Source: three-view drawing plus pictorial views. Frame: mm from the lowest corner of the part. A direction names the side the tool comes from. Give positions to 0.01 mm unless a question says otherwise; leave off trailing zeros. Loops run counter-clockwise (first coordinate to the right, second up) from the corner with the lowest first, then second, coordinate; pieces in that order, holes last. Notation, with made-up numbers: (-16.75, -11) - (37.25, -11) arc R12 cw to (37.25, 10) - close; hole circle Ø11 at (8, 2). An arc over 180 degrees is marked (long way). Answer as a JSON object with one key per item and string values. Group by question number.
(1) Material intervals for L1, parallel to Z at x = 3.5, y = 18.25; L2, parallel to X at y = 12, z = 20; L3, parallel to X at y = 17.5, z = 14.75 (3 decimals), sorted ascending.
(2) Section query B-B (z = 8). Return loops of the section in (x, y), plus the area to 3 significant figures.
(3) Pin query (flat end, axial travel): P1, Ø8, axis at x = 42, y = 12, coming from the +Z side; P2, Ø1, axis at x = 17.5, y = 10, coming from the +Z side; P3, Ø10, axis at y = 10, z = 16.5, coming from the -X side. Return the tip coordinate at first contact, or that it passes through.
(4) Section query C-C (x = 27.5). Return loops of the section in (y, z).
(5) Access query for the marked faces 1 and 2. Directions: +Z, -Z, +X, -X, +Y, -Y. A direction counts if a zero-diameter tool reaches every point of the face in a straight line with its end or side. Return the directions, or none.
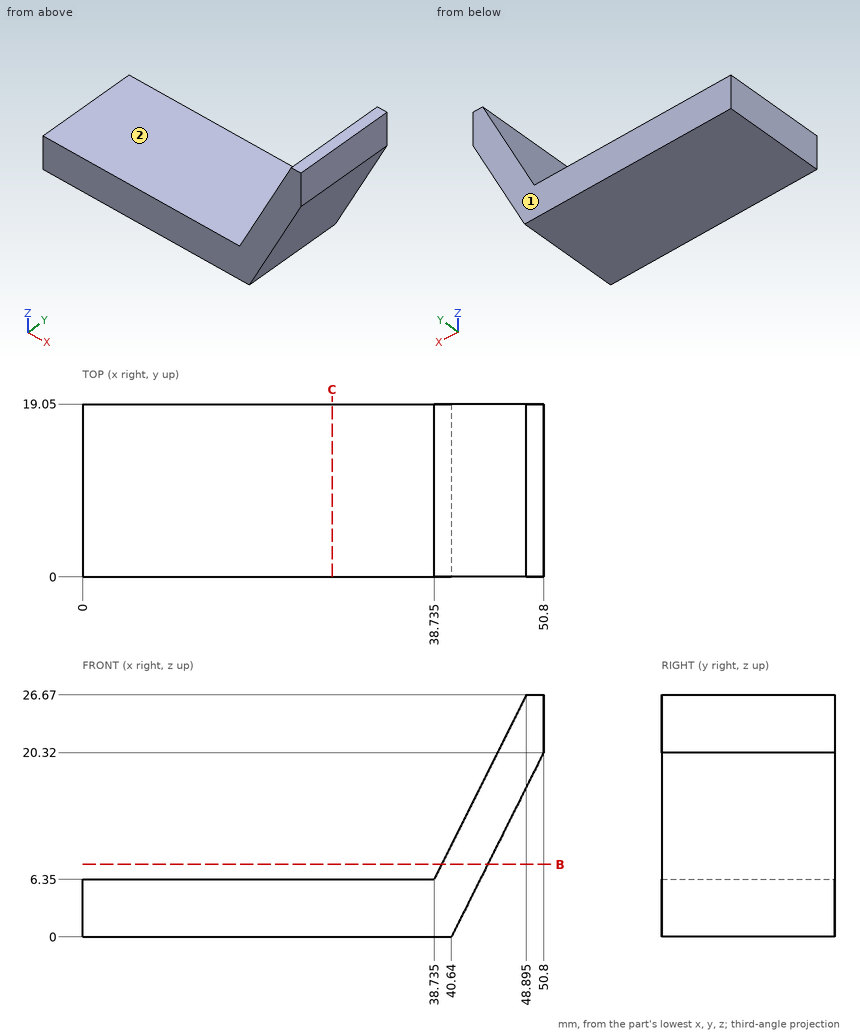
Recorded:
{
 "1": {"L1": "z = 0 to 6.35", "L2": "x = 45.56 to 50.64", "L3": "x = 42.935 to 48.015"},
 "2": {"outline": "(39.56, 0) - (44.64, 0) - (44.64, 19.05) - (39.56, 19.05) - close", "area": "96.8 mm^2"},
 "3": {"P1": "stops at z = 20.88", "P2": "stops at z = 6.35", "P3": "stops at x = 41.31"},
 "4": {"outline": "(0, 0) - (19.05, 0) - (19.05, 6.35) - (0, 6.35) - close"},
 "5": {"face 1": "+Z, -Z, +X, -X, +Y", "face 2": "+Z, -X, +Y, -Y"}
}
